Here's how the part is built. I have some questions about the finished solid (model axes, mm). Face numbers are marked on the shaded views. A direction names the side the tool comes from. Coordinates: 2 decimals unless noted, no trailing zeros. Write each loop counter-clockwise with the first axis right and the second up, starting at its lowest first coordinate (ties: lowest second). Pieces come first, ordered by that corner, then holes.
Item 1: If we section it at A-A (y = 0): Please give me the cut outline in (x, z), then the cut area to 3 significant figures.
Item 2: For the marked faces 1, 2 and 3, which set-ups out of +Z, -Z, +X, -X, +Y, -Y let a thin tool reach every point of the face, with its end or its side?
Item 3: If we section it at B-B (z = 29): Please give me the cut outline in (x, y), then the cut area to 3 significant figures.
Item 4: If I drill on line 1 (Y direction, x = -34.8, z = 58.5); line 2 (Z direction, x = 9, y = -9.5); line 3 (Z direction, x = 36, y = -10), over which ranges is the centre line in solid material (lowest first)?
Item 5: I'm going to push flat-ended pins straight in: pin 1 Ø10 at (x, y) = (32.5, -33) entering from +Z; pin 2 Ø1 at (x, y) = (-30, -13.5) entering from +Z; pin 3 Ø4 at (y, z) = (-40.5, -26) entering from +X. Where does each tip first touch, or does it pass through?
Item 6: If we section it at D-D (x = 9): Please give me the cut outline in (y, z).
from build123d import *

# Parameters (mm, degrees)
SKETCH_3_W               = 86
SKETCH_3_H               = 86
EXTRUDE_2_DEPTH          = 64.5
CUT_EXTRUDE_2_DEPTH      = 106
PATTERN_CIRCULAR_1_COUNT = 4
SKETCH_5_R               = 2.75
CUT_EXTRUDE_3_DEPTH      = 10
SKETCH_6_R               = 36.5
EXTRUDE_3_DEPTH          = 1.5
SKETCH_7_R               = 6.35
EXTRUDE_4_DEPTH          = 30


with BuildPart() as part:
    # Sketch 3 → Extrude 2 (new body, symmetric)
    with BuildSketch(Plane.XY):
        Rectangle(SKETCH_3_W, SKETCH_3_H)
    extrude(amount=EXTRUDE_2_DEPTH, both=True)

    # Sketch 4 → Cut-Extrude 2 (cut)
    with BuildSketch(Plane(origin=(0, 0, -64.5), x_dir=(-1, 0, 0), z_dir=(0, 0, -1))):
        with BuildLine():
            Line((-28.8, 34.8), (-28.8, 43))
            Line((-28.8, 43), (-43, 43))
            Line((-43, 43), (-43, 28.8))
            Line((-43, 28.8), (-34.8, 28.8))
            ThreePointArc((-34.8, 28.8), (-30.557359313, 30.557359313), (-28.8, 34.8))
        make_face()
    cut_extrude_2 = extrude(amount=-CUT_EXTRUDE_2_DEPTH, mode=Mode.SUBTRACT)

    # Pattern Circular 1: Cut-Extrude 2 ×4 about axis
    pattern_circular_1_axis = Axis((0, 0, 0), (0, 0, 1))
    for i in range(1, PATTERN_CIRCULAR_1_COUNT):
        add(cut_extrude_2.rotate(pattern_circular_1_axis, i * 360 / PATTERN_CIRCULAR_1_COUNT), mode=Mode.SUBTRACT)

    # Sketch 5 → Cut-Extrude 3 (cut)
    with BuildSketch(Plane.XY.offset(64.5)):
        with Locations((-34.8, 34.8)):
            Circle(SKETCH_5_R)
        with Locations((35.2, 34.8)):
            Circle(SKETCH_5_R)
        with Locations((35.2, -35.2)):
            Circle(SKETCH_5_R)
        with Locations((-34.8, -35.2)):
            Circle(SKETCH_5_R)
    extrude(amount=-CUT_EXTRUDE_3_DEPTH, mode=Mode.SUBTRACT)

    # Sketch 6 → Extrude 3 (add)
    with BuildSketch(Plane.XY.offset(64.5)):
        Circle(SKETCH_6_R)
    extrude(amount=EXTRUDE_3_DEPTH)

    # Sketch 7 → Extrude 4 (add)
    with BuildSketch(Plane.XY.offset(66)):
        Circle(SKETCH_7_R)
    extrude(amount=EXTRUDE_4_DEPTH)


solid = part.part
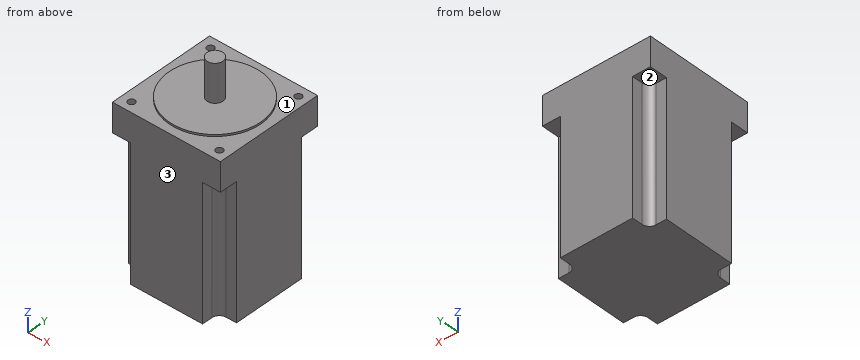
Answer list:
1. outline: (-43, -64.5) - (43, -64.5) - (43, 64.5) - (36.5, 64.5) - (36.5, 66) - (6.35, 66) - (6.35, 96) - (-6.35, 96) - (-6.35, 66) - (-36.5, 66) - (-36.5, 64.5) - (-43, 64.5) - close
1. area: 11,600 mm2
2. face 1: +Z
2. face 2: -Z, -X, +Y
2. face 3: +Z, -Z, +X, -X, -Y
3. outline: (-43, -28.8) - (-34.8, -28.8) arc R6 cw to (-28.8, -34.8) - (-28.8, -43) - (28.8, -43) - (28.8, -34.8) arc R6 cw to (34.8, -28.8) - (43, -28.8) - (43, 28.8) - (34.8, 28.8) arc R6 cw to (28.8, 34.8) - (28.8, 43) - (-28.8, 43) - (-28.8, 34.8) arc R6 cw to (-34.8, 28.8) - (-43, 28.8) - close
3. area: 6,620 mm2
4. line 1: y = -43 to -37.95, -32.45 to 32.05, 37.55 to 43
4. line 2: z = -64.5 to 66
4. line 3: z = -64.5 to 64.5
5. pin 1: stops at z = 64.5
5. pin 2: stops at z = 66
5. pin 3: stops at x = 28.8
6. outline: (-43, -64.5) - (43, -64.5) - (43, 64.5) - (35.37, 64.5) - (35.37, 66) - (-35.37, 66) - (-35.37, 64.5) - (-43, 64.5) - close
